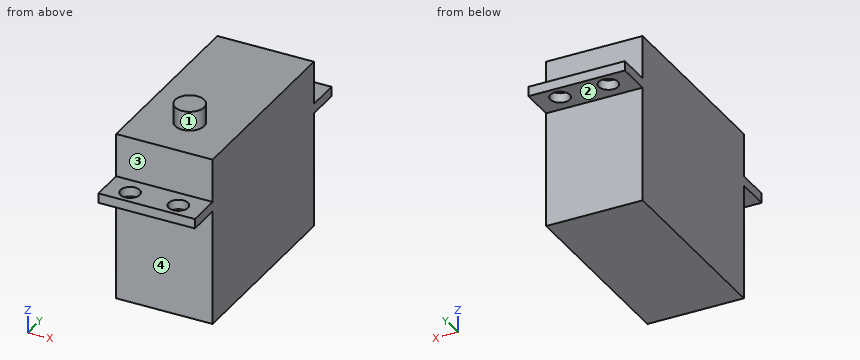
```python
from build123d import *

# Parameters (mm, degrees)
F0_W     = 20
F0_H     = 7
F0_R     = 2
F0_H_2   = 40
F1_DEPTH = 2
F2_DEPTH = 11
F3_DEPTH = 24
F4_R     = 3
F5_DEPTH = 4


with BuildPart() as f1:
    # F0 (on Top) → F1 (new body)
    with BuildSketch(Plane.XY):
        with Locations((10, 50.5)):
            Rectangle(F0_W, F0_H)
        with Locations((5, 51)):
            Circle(F0_R, mode=Mode.SUBTRACT)
        with Locations((15, 51)):
            Circle(F0_R, mode=Mode.SUBTRACT)
        with Locations((10, 27)):
            Rectangle(F0_W, F0_H_2)
        with Locations((10, 3.5)):
            Rectangle(F0_W, F0_H)
        with Locations((5, 3)):
            Circle(F0_R, mode=Mode.SUBTRACT)
        with Locations((15, 3)):
            Circle(F0_R, mode=Mode.SUBTRACT)
    extrude(amount=F1_DEPTH)

    # F0 (on Top) → F2 (join)
    with BuildSketch(Plane.XY):
        with Locations((10, 27)):
            Rectangle(F0_W, F0_H_2)
    extrude(amount=F2_DEPTH)

    # F0 (on Top) → F3 (join)
    with BuildSketch(Plane.XY):
        with Locations((10, 27)):
            Rectangle(F0_W, F0_H_2)
    extrude(amount=-F3_DEPTH)

    # F4 (on face) → F5 (join)
    with BuildSketch(Plane.XY.offset(11)):
        with Locations((10, 17)):
            Circle(F4_R)
    extrude(amount=F5_DEPTH)


solid = f1.part
```
Model file for the job. Use its own axes, mm. Face numbers are marked on the shaded views. A direction names the side the tool comes from. Coordinates: 2 decimals unless noted, no trailing zeros. Write each loop counter-clockwise with the first axis right and the second up, starting at its lowest first coordinate (ties: lowest second). Pieces come first, ordered by that corner, then holes. Notation, with made-up numbers: (58.25, -28) - (99.25, -28) arc R13 ccw to (99.25, -22) - close; hole circle Ø7 at (-38.75, 1). An arc over 180 degrees is marked (long way). One line per question, with ' | ' between items. Start each with the question number.
Q1. Cut at D-D, the plane x = 11. List the corners of the cut face in (y, z).
Q2. Pin check, flat tips, straight feed: pin 1 (2 mm diameter, centred on y = 7.5, z = -7.5, fed in from -X); pin 2 (1.5 mm diameter, centred on x = 15.5, z = 4, fed in from +Y); pin 3 (4 mm diameter, centred on x = 4, y = 47.5, fed in from +Z); pin 4 (2 mm diameter, centred on x = 12.5, y = 49, fed in from -Z). Stop position of each tip, or through.
Q3. Cut at B-B, the plane x = 5. List the corners of the cut face in (y, z).
Q4. Drill centre lines: line 1 (Y direction, x = 15, z = 0.7); line 2 (Z direction, x = 13.5, y = 21); line 3 (Y direction, x = 9, z = -19). Where is each one in solid material? Low to high. Write a range as [from, to].
Q5. Cut at C-C, the plane y = 17. List the corners of the cut face in (x, z), then the cut area to 3 significant figures.
Q6. 3-axis set-ups, long thin cutter, end or side, ignore diameter. For the marked faces 1, 2, 3 and 4: which of +Z, -Z, +X, -X, +Y, -Y reach the whole face in a straight line?
Q7. Cut at A-A, the plane y = 51. List the corners of the cut face in (x, z), then the cut area to 3 significant figures.
Answer below:
1) outline: (0, 0) - (7, 0) - (7, -24) - (47, -24) - (47, 0) - (54, 0) - (54, 2) - (47, 2) - (47, 11) - (19.83, 11) - (19.83, 15) - (14.17, 15) - (14.17, 11) - (7, 11) - (7, 2) - (0, 2) - close
2) pin 1: x = 0 | pin 2: y = 47 | pin 3: z = 11 | pin 4: z = 0
3) outline: (0, 0) - (1, 0) - (1, 2) - (0, 2) - close; (5, 0) - (7, 0) - (7, -24) - (47, -24) - (47, 0) - (49, 0) - (49, 2) - (47, 2) - (47, 11) - (7, 11) - (7, 2) - (5, 2) - close; (53, 0) - (54, 0) - (54, 2) - (53, 2) - close
4) line 1: [0, 1], [5, 49], [53, 54] | line 2: [-24, 11] | line 3: [7, 47]
5) outline: (0, -24) - (20, -24) - (20, 11) - (13, 11) - (13, 15) - (7, 15) - (7, 11) - (0, 11) - close | area: 724 mm^2
6) face 1: +Z | face 2: -Z, +X, -X, +Y | face 3: +Z, +X, -X, -Y | face 4: -Z, +X, -X, -Y
7) outline: (0, 0) - (3, 0) - (3, 2) - (0, 2) - close; (7, 0) - (13, 0) - (13, 2) - (7, 2) - close; (17, 0) - (20, 0) - (20, 2) - (17, 2) - close | area: 24.0 mm^2
